The model under review builds one solid part; all positions refer to its coordinate system, in mm. A direction names the side the tool comes from. Coordinates: 2 decimals unless noted, no trailing zeros. Write each loop counter-clockwise with the first axis right and the second up, starting at its lowest first coordinate (ties: lowest second). Pieces come first, ordered by that corner, then holes. Notation, with made-up numbers: M -33.75,58.25 L -24.75,58.25 A4 ccw -24.75,62.25 Z; hole C 89,54 d7. An arc over 180 degrees is marked long. Answer as a JSON object with one key per item and string values.
```python
from build123d import *

# Parameters (mm, degrees)
F0_R            = 79
F0_R_2          = 33
F1_DEPTH        = 20
F2_R            = 67.075
F3_DEPTH        = 13
F4_SIZE         = 5
F6_DEPTH        = 20.001
F6_COPIES_COUNT = 5


# Not quite as in the source:
# - a pattern or mirror of a feature is missing from the dataset's text; its kind, count and spacing are read off the source's solid


with BuildPart() as f1:
    # F0 (on Front) → F1 (new body)
    with BuildSketch(Plane.XZ):
        Circle(F0_R)
        Circle(F0_R_2, mode=Mode.SUBTRACT)
    extrude(amount=F1_DEPTH)

    # F2 (on face) → F3 (cut)
    with BuildSketch(Plane.XZ.offset(20)):
        Circle(F2_R)
    extrude(amount=-F3_DEPTH, mode=Mode.SUBTRACT)

    # F4
    f4_edges = [f1.edges().sort_by_distance(p)[0] for p in [
        (-33, -7, 0),
    ]]
    chamfer(f4_edges, length=F4_SIZE)

    # F5 (on face) → F6 (cut, through all)
    with BuildSketch(Plane.XZ.offset(20)):
        with BuildLine():
            ThreePointArc((-7.4875080879, 64.5673076923), (0, 57.5), (7.4875080879, 64.5673076923))
            ThreePointArc((7.4875080879, 64.5673076923), (0, 65), (-7.4875080879, 64.5673076923))
        make_face()
        with BuildLine():
            ThreePointArc((-7.4875080879, 64.5673076923), (0, 65), (7.4875080879, 64.5673076923))
            ThreePointArc((7.4875080879, 64.5673076923), (7.4968763715, 64.7835637039), (7.5, 65))
            ThreePointArc((7.5, 65), (7.4524663535, 65.843057086), (7.3104679333, 66.6754278846))
            ThreePointArc((7.3104679333, 66.6754278846), (0, 67.075), (-7.3104679333, 66.6754278846))
            ThreePointArc((-7.3104679333, 66.6754278846), (-7.4736916091, 65.6276414045), (-7.4875080879, 64.5673076923))
        make_face()
        with BuildLine():
            ThreePointArc((7.3104679333, 66.6754278846), (0, 72.5), (-7.3104679333, 66.6754278846))
            ThreePointArc((-7.3104679333, 66.6754278846), (0, 67.075), (7.3104679333, 66.6754278846))
        make_face()
    f6 = extrude(amount=-F6_DEPTH, mode=Mode.SUBTRACT)

    # F6_copies: F6 ×5 about axis
    f6_copies_axis = Axis((0, 0, 0), (0, 1, 0))
    for i in range(1, F6_COPIES_COUNT):
        add(f6.rotate(f6_copies_axis, i * 360 / F6_COPIES_COUNT), mode=Mode.SUBTRACT)


solid = f1.part
```
(1) Add section C-C on x = 0. Give the boundary of the cut face in (y, z) (3 decimals).
Results list:
{"outline": "M -20,-79 L 0,-79 L 0,-33 L -2,-33 L -7,-38 L -7,-67.075 L -20,-67.075 Z; M -20,72.5 L 0,72.5 L 0,79 L -20,79 Z; M -7,38 L -2,33 L 0,33 L 0,57.5 L -7,57.5 Z"}
(2) Wall thickness on line 1 along Z through (x, y) = (0, -1.3); line 2 along Y through (x, z) = (-42, -29.5); line 3 along X through (y, z) = (-9, -11.5): over which ranges is each line inside the solid? List them lowest first. Write a range as from..to.
Results list:
{"line 1": "-79..-33, 33..57.5, 72.5..79", "line 2": "-7..0", "line 3": "-78.16..-66.08, 66.08..78.16"}
(3) Add section A-A on z = 0. Give the boundary of the cut face in (x, y) (3 decimals), and give its area (3 significant figures).
Results list:
{"outline": "M -79,-20 L -67.075,-20 L -67.075,-7 L -38,-7 L -33,-2 L -33,0 L -79,0 Z; M 33,-2 L 38,-7 L 67.075,-7 L 67.075,-20 L 79,-20 L 79,0 L 33,0 Z", "area": "929 mm²"}
(4) For pin 1 Ø2 at (x, y) = (-10.5, -7) entering from +Z; pin 2 Ø2 at (y, z) = (-16.5, 53) entering from -X; pin 3 Ø6 at (y, z) = (-16.5, -58.5) entering from +X, all flat-tipped, find the tip position at first contact; note any pin that passes through.
Results list:
{"pin 1": "z = 78.43", "pin 2": "x = -59.47", "pin 3": "x = 56.22"}
(5) Draft analysis for pull direction X (two halves, no side actions). For faces 3 (the face through (-58.23, -9.86, 53.39)), 4 (the face through (39.819, -13.591, 53.977)), 5 (the face through (-1, 0, -34)), state which applies: released by +X, released by -X, zero draft, split by the parting line, or undercut.
Results list:
{"face 3": "split by the parting line", "face 4": "undercut", "face 5": "zero draft"}
(6) Add section D-D on y = -4.25. Count the separate pieces of the cut face and the enclosed holes in it, and give its area (3 significant figures).
Results list:
{"separate pieces": "1", "enclosed holes": "6", "area": "14,800 mm²"}
(7) For faces 1 (the face through (30.5, -1, -12.6)), 2 (the face through (-63.94, -13.59, -20.26)), list the 3-axis set-ups (+Z, -Z, +X, -X, +Y, -Y) from which the entire face can be reached by the end or side of a thin tool; tool diameter is ignored.
Results list:
{"face 1": "+Y, -Y", "face 2": "-Y"}
